For this review, take the finished solid that the model builds, in its own axes (mm). A direction names the side the tool comes from. Round coordinates to 2 decimals unless told otherwise and drop trailing zeros. Order: outer loops, then holes, each group sorted by start corner. A loop starts at its lowest first (then second) coordinate and runs counter-clockwise, first axis right, second up. Notation, with made-up numbers: (74.5, -17.75) -> (80.5, -17.75) arc R12 cw to (80.5, -10.75) -> close; hole circle Ø11 at (14.25, 21). An arc over 180 degrees is marked (long way). Use a Markdown table: item, result. Add a question column.
1) Consider section D-D (y = -42.5). State the section outline as (x, z) points.
2) Machinability: for faces 1 (the face through (3, 0, 3)), 2 (the face through (0.056, -7.791, -11.988)), 3 (the face through (-2.03, 6.48, -1.89)), 4 (the face through (0, -57, -3)), which of the approach directions +Z, -Z, +X, -X, +Y, -Y give a long, thin tool a straight path to every point of the face, cutting with its end or side? Answer none if there is none.
3) Consider section C-C (z = -6.5). State the section outline as (x, y) points.
4) Draft analysis for pull direction Y (two halves, no side actions). For faces 5 (the face through (1.969, 8.172, -7.645)), 6 (the face through (0, -95, -8)), 7 (the face through (4, -32, -6)), 8 (the face through (1.911, 25.807, -10.618)), state which applies: pulls with the +Y half, pulls with the -Y half, needs draft (parallel to the pull), parting line crosses it, or undercut.
5) Clearance check with flat-ended pins moving along their axes: P1, Ø4, axis at x = 2, y = -15.5, coming from the -Z side; P2, Ø1.5, axis at x = 0, y = -35.5, coming from the +Z side; P3, Ø4.5, axis at y = 25.37, z = -9.23, coming from the -X side. State where each tip first meets the part, or that it passes through.
6) Wall thickness on line 1 along Z through (x, y) = (2.75, -40); line 2 along Z through (x, y) = (2.75, -0.5); line 3 along Z through (x, y) = (2, 13): over which ranges is each line inside the solid? List them lowest first. Write a range as [from, to].
```python
from build123d import *

# Parameters (mm, degrees)
SKETCH1_R           = 2.5
SKETCH1_R_2         = 1.45
BOSS_EXTRUDE1_DEPTH = 4
SKETCH2_R           = 3
CUT_EXTRUDE1_DEPTH  = 3.3
CUT_EXTRUDE2_START  = -0.12
SKETCH1_5_R         = 4.5
SKETCH1_5_R_2       = 1.45
CUT_EXTRUDE2_DEPTH  = 96.951003405
CUT_EXTRUDE3_START  = -5.7
SKETCH2_2_R         = 3
CUT_EXTRUDE3_DEPTH  = 2.3
CHAMFER1_SIZE2      = 0.5
CHAMFER1_SIZE       = 1


with BuildPart() as part:
    # Sketch1 → Boss-Extrude1 (new, symmetric)
    with BuildSketch(Plane(origin=(0, 0, 0), x_dir=(0, 0, -1), z_dir=(1, 0, 0))):
        with BuildLine():
            Line((3, -24), (3, -90))
            ThreePointArc((3, -90), (8, -95), (13, -90))
            Line((13, -90), (13, -17.799320055))
            ThreePointArc((13, -17.799320055), (11.959160872, -7.650400571), (8.879977332, 2.075983213))
            ThreePointArc((8.879977332, 2.075983213), (7.645623758, 8.261271435), (9.063072492, 14.407185379))
            Line((9.063072492, 14.407185379), (13.308813282, 23.461117406))
            ThreePointArc((13.308813282, 23.461117406), (10.999511856, 29.511131641), (5.035153889, 26.988835198))
            Line((5.035153889, 26.988835198), (-4.665988868, 1.79681604))
            ThreePointArc((-4.665988868, 1.79681604), (-4.952494502, -0.687603231), (-4, -3))
            ThreePointArc((-4, -3), (1.203915432, -12.932028189), (3, -24))
        make_face()
        Circle(SKETCH1_R, mode=Mode.SUBTRACT)
        with Locations((9.23454387, 25.371700761)):
            Circle(SKETCH1_R_2, mode=Mode.SUBTRACT)
    extrude(amount=BOSS_EXTRUDE1_DEPTH, both=True)

    # Sketch2 → Cut-Extrude1 (cut)
    with BuildSketch(Plane(origin=(4, 0, 0), x_dir=(0, 0, -1), z_dir=(1, 0, 0))):
        Circle(SKETCH2_R)
    extrude(amount=-CUT_EXTRUDE1_DEPTH, mode=Mode.SUBTRACT)

    # Sketch1<5> → Cut-Extrude2 (cut, through all)
    # profile 1 of 2: a face of its own
    with BuildSketch(Plane(origin=(0, 0, 0), x_dir=(0, 0, -1), z_dir=(1, 0, 0)).offset(CUT_EXTRUDE2_START)):
        with BuildLine():
            ThreePointArc((-4.665988868, 1.79681604), (2.013271717, 6.484076223), (8.879977332, 2.075983213))
            ThreePointArc((8.879977332, 2.075983213), (7.645623758, 8.261271435), (9.063072492, 14.407185379))
            Line((9.063072492, 14.407185379), (13.308813282, 23.461117406))
            ThreePointArc((13.308813282, 23.461117406), (7.469575883, 21.232269882), (5.035153889, 26.988835198))
            Line((5.035153889, 26.988835198), (-4.665988868, 1.79681604))
        make_face()
    # profile 2 of 2: a face of its own
    with BuildSketch(Plane(origin=(0, 0, 0), x_dir=(0, 0, -1), z_dir=(1, 0, 0)).offset(CUT_EXTRUDE2_START)):
        with Locations((9.23454387, 25.371700761)):
            Circle(SKETCH1_5_R)
        with Locations((9.23454387, 25.371700761)):
            Circle(SKETCH1_5_R_2, mode=Mode.SUBTRACT)
    extrude(amount=-CUT_EXTRUDE2_DEPTH, mode=Mode.SUBTRACT)

    # Sketch2<2> → Cut-Extrude3 (cut)
    with BuildSketch(Plane(origin=(4, 0, 0), x_dir=(0, 0, -1), z_dir=(1, 0, 0)).offset(CUT_EXTRUDE3_START)):
        Circle(SKETCH2_2_R)
    extrude(amount=-CUT_EXTRUDE3_DEPTH, mode=Mode.SUBTRACT)

    # Chamfer1
    chamfer1_edges = [part.edges().sort_by_distance(p)[0] for p in [
        (0.7, 0, 3),
    ]]
    chamfer1_side = [part.faces().sort_by_distance(p)[0] for p in [
        (0.71, 0, 3),
    ]]
    chamfer(chamfer1_edges, length=CHAMFER1_SIZE - 0.0001, length2=CHAMFER1_SIZE2 - 0.0001, reference=chamfer1_side[0])  # a hair under: the kernel refuses the full size


solid = part.part
```
Results list:
| question | item | result |
|---|---|---|
| 1 | outline | (-4, -13) -> (4, -13) -> (4, -3) -> (-4, -3) -> close |
| 2 | face 1 | +X |
| 2 | face 2 | -Z, +X, -X |
| 2 | face 3 | -X, +Y |
| 2 | face 4 | +Z, +X, -X, -Y |
| 3 | outline | (-4, -94.77) -> (4, -94.77) -> (4, 28.95) -> (-0.12, 28.95) -> (-0.12, 5.06) -> (-4, 5.06) -> close |
| 4 | face 5 | undercut |
| 4 | face 6 | pulls with the -Y half |
| 4 | face 7 | needs draft |
| 4 | face 8 | undercut |
| 5 | P1 | z = -13 |
| 5 | P2 | z = -3 |
| 5 | P3 | x = -0.12 |
| 6 | line 1 | [-13, -3] |
| 6 | line 2 | [-9.91, -2.96], [2.96, 4.97] |
| 6 | line 3 | [-8.49, 0.35] |
